```python
from build123d import *

# Parameters (mm, degrees)
F1_W      = 48
F1_H      = 36
F2_DEPTH  = 1.5
F4_W      = 42
F4_H      = 30.5
F4_W_2    = 39
F4_H_2    = 27.5
F6_DEPTH  = 0.7
F7_R      = 2
F8_R      = 1
F9_DEPTH  = 25
F10_SIZE2 = 0.9
F10_SIZE  = 0.9
F11_R     = 2


with BuildPart() as f2:
    # F1 (on Top) → F2 (new body)
    with BuildSketch(Plane.XY):
        with Locations((19, 13.25)):
            Rectangle(F1_W, F1_H)
    extrude(amount=F2_DEPTH)

    # F4 (on face) → F6 (cut)
    with BuildSketch(Plane.XY.offset(1.5)):
        with Locations((19, 13.25)):
            Rectangle(F4_W, F4_H)
        with Locations((19, 13.25)):
            Rectangle(F4_W_2, F4_H_2, mode=Mode.SUBTRACT)
    extrude(amount=-F6_DEPTH, mode=Mode.SUBTRACT)

    # F7
    f7_edges = [f2.edges().sort_by_distance(p)[0] for p in [
        (40, 28.5, 1.15),
        (40, -2, 1.15),
        (-2, 28.5, 1.15),
        (-2, -2, 1.15),
    ]]
    fillet(f7_edges, radius=F7_R)

    # F8
    f8_edges = [f2.edges().sort_by_distance(p)[0] for p in [
        (38.5, 27, 1.15),
        (38.5, -0.5, 1.15),
        (-0.5, -0.5, 1.15),
        (-0.5, 27, 1.15),
    ]]
    fillet(f8_edges, radius=F8_R)

    # F5 (on face) → F9 (cut)
    with BuildSketch(Plane.XY.offset(1.5)):
        with BuildLine():
            Line((40, 28.5), (39.6632503002, 28.5))
            ThreePointArc((39.6632503002, 28.5), (39.7993596875, 28.2508547004), (40, 28.05))
            Line((40, 28.05), (40, 28.5))
        make_face()
        with BuildLine():
            ThreePointArc((41.6, 28.85), (40.4221653855, 29.8340603893), (39.6632503002, 28.5))
            Line((39.6632503002, 28.5), (40, 28.5))
            Line((40, 28.5), (40, 28.05))
            ThreePointArc((40, 28.05), (41.0472135955, 27.955572809), (41.6, 28.85))
        make_face()
    extrude(amount=-F9_DEPTH, mode=Mode.SUBTRACT)

    # F10
    f10_edges = [f2.edges().sort_by_distance(p)[0] for p in [
        (41.2, 29.65, 0),
    ]]
    chamfer(f10_edges, length=F10_SIZE, length2=F10_SIZE2)

    # F11
    f11_edges = [f2.edges().sort_by_distance(p)[0] for p in [
        (43, 31.25, 0.75),
    ]]
    fillet(f11_edges, radius=F11_R)


solid = f2.part
```
The listing builds one solid part. Answer for the finished solid, in the listing's coordinates (mm). A direction names the side the tool comes from. Give positions to 0.01 mm unless a question says otherwise; leave off trailing zeros. Loops run counter-clockwise (first coordinate to the right, second up) from the corner with the lowest first, then second, coordinate; pieces in that order, holes last. Notation, with made-up numbers: M 85.25,-2.5 L 89.25,-2.5 A25 ccw 89.25,21.5 Z; hole C 39.25,-31.5 d1. An arc over 180 degrees is marked long. One line per item, written item: value.
1. This flat-tipped pin is pushed along its axis until it touches: P1, Ø3, axis at x = 40.6, y = 28.85, coming from the -Z side. Where does it stop, or does it pass through?
Found:
P1: z = 0.4
2. For faces 4 (the face through (43, 12, 1)), 5 (the face through (-1.4, 27.93, 1.15)), determine the directions among +Z, -Z, +X, -X, +Y, -Y from which every point of the face is accessible in a straight line to the end or side of a thin tool.
Found:
face 4: +Z, -Z, +X, +Y, -Y
face 5: +Z
3. Find the intervals of material crossed by probe 1 along Y at (x, z) = (4.5, 0.95); probe 2 along X at (y, z) = (25.5, 0.85); probe 3 along Y at (x, z) = (40.6, 1.25), in increasing order.
Found:
probe 1: -4.75 to -2, -0.5 to 27, 28.5 to 31.25
probe 2: -5 to -2, -0.5 to 38.5, 40 to 43
probe 3: -4.75 to 27.85, 29.85 to 31.25
4. For a pull along Y with two mould halves and no side action, classify faces 1 (the face through (38.199, -0.215, 1.145)), 2 (the face through (18, 31.25, 1)), 3 (the face through (21, 29, 1.5)) as pulls with the +Y half, pulls with the -Y half, needs draft (parallel to the pull), parting line crosses it, or undercut.
Found:
face 1: undercut
face 2: pulls with the +Y half
face 3: needs draft
5. Section B-B on x = 2.5 is taken. Determine the outline of the cut face in (y, z).
Found:
outline: M -4.75,0 L 31.25,0 L 31.25,1.5 L 28.5,1.5 L 28.5,0.8 L 27,0.8 L 27,1.5 L -0.5,1.5 L -0.5,0.8 L -2,0.8 L -2,1.5 L -4.75,1.5 Z
6. Section A-A on y = 15 is taken. Determine the outline of the cut face in (x, z), plus the area to 3 significant figures.
Found:
outline: M -5,0 L 43,0 L 43,1.5 L 40,1.5 L 40,0.8 L 38.5,0.8 L 38.5,1.5 L -0.5,1.5 L -0.5,0.8 L -2,0.8 L -2,1.5 L -5,1.5 Z
area: 69.9 mm^2
